Verification items for this drawing (mm, ordinates from the low corner). A direction names the side the tool comes from. Coordinates: 2 decimals unless noted, no trailing zeros. Write each loop counter-clockwise with the first axis right and the second up, starting at its lowest first coordinate (ties: lowest second). Pieces come first, ordered by that corner, then holes. Notation, with made-up numbers: M 29,-5.75 L 83,-5.75 A9 ccw 83,3.25 Z; hole C 39,32 d10. An arc over 180 degrees is marked long. Answer as CSV lines item,"result". Start each with the question number.
1) Go/stop test with flat-tipped pins: pin 1 Ø1 at (x, z) = (19.5, 23) entering from +Y; pin 2 Ø1.5 at (y, z) = (5.5, 24.5) entering from -X; pin 3 Ø1 at (x, z) = (17, 18.5) entering from +Y. Record where each tip stops, or that it passes through.
2) Section check C-C (z = 27). Record the cut outline in (x, y), and give its area (3 significant figures).
3) Access from +Z, -Z, +X, -X, +Y, -Y to the whole of each face (thin tool, end or side, straight path). Record for the marked faces 1 and 2.
4) Section check A-A (x = 12.2). Record the cut outline in (y, z), and give its area (3 significant figures).
5) Material ranges on L1, parallel to Z at x = 5.25, y = 9.75; L2, parallel to Y at x = 19.5, z = 16 (1 decimal); L3, parallel to X at y = 17.75, z = 18 (1 decimal), recorded low to high. Write a range as [from, to].
6) Section check B-B (y = 12.2). Record the cut outline in (x, z), and give its area (3 significant figures).
7) Section check D-D (y = 2.95). Record the cut outline in (x, z) (1 decimal), and give its area (3 significant figures).
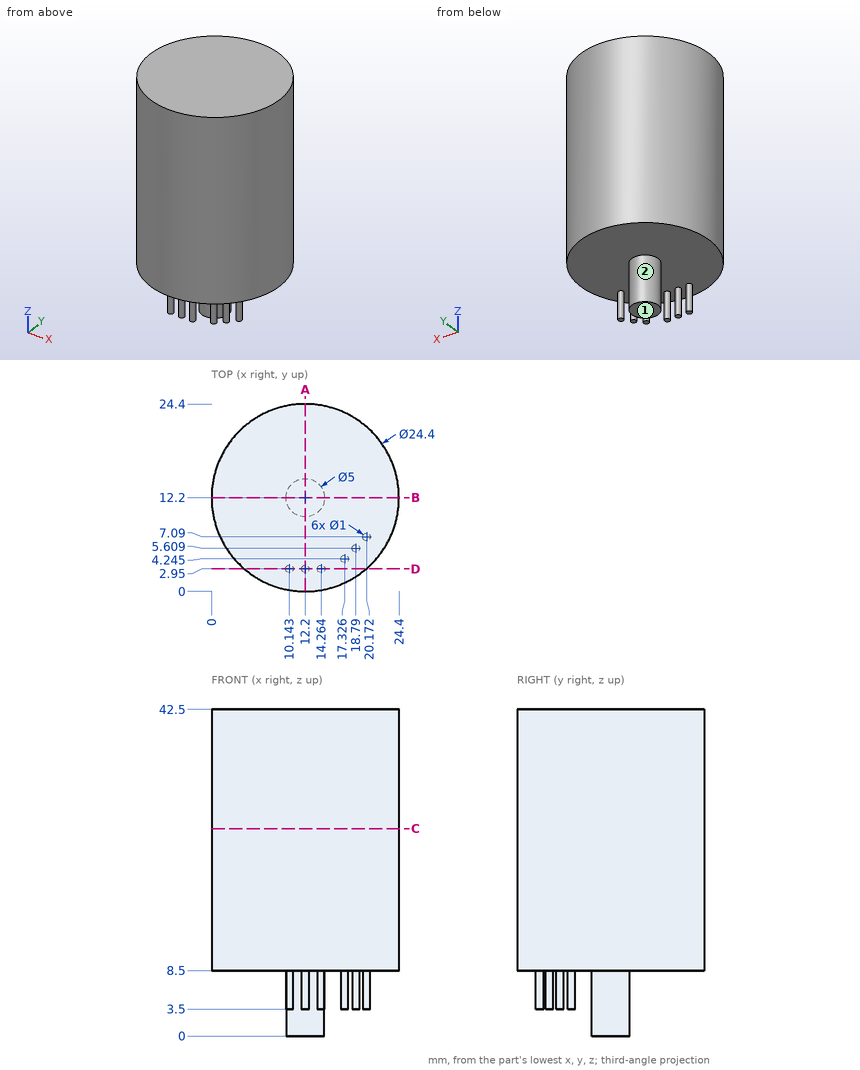
Results found:
1,pin 1,"stops at y = 22.33"
1,pin 2,"stops at x = 1.55"
1,pin 3,"stops at y = 23.62"
2,outline,"C 12.2,12.2 d24.4"
2,area,"468 mm2"
3,face 1,"-Z, +X, -X, +Y, -Y"
3,face 2,"-Z"
4,outline,"M 0,8.5 L 2.45,8.5 L 2.45,3.5 L 3.45,3.5 L 3.45,8.5 L 9.7,8.5 L 9.7,0 L 14.7,0 L 14.7,8.5 L 24.4,8.5 L 24.4,42.5 L 0,42.5 Z"
4,area,"877 mm2"
5,L1,"z = [8.5, 42.5]"
5,L2,"y = [2.4, 22]"
5,L3,"x = [1.3, 23.1]"
6,outline,"M 0,8.5 L 9.7,8.5 L 9.7,0 L 14.7,0 L 14.7,8.5 L 24.4,8.5 L 24.4,42.5 L 0,42.5 Z"
6,area,"872 mm2"
7,outline,"M 4.2,8.5 L 9.6,8.5 L 9.6,3.5 L 10.6,3.5 L 10.6,8.5 L 11.7,8.5 L 11.7,3.5 L 12.7,3.5 L 12.7,8.5 L 13.8,8.5 L 13.8,3.5 L 14.8,3.5 L 14.8,8.5 L 20.2,8.5 L 20.2,42.5 L 4.2,42.5 Z"
7,area,"556 mm2"
